Here's how the part is built. I have some questions about the finished solid (model axes, mm). Give positions to 0.01 mm unless a question says otherwise; leave off trailing zeros. Loops run counter-clockwise (first coordinate to the right, second up) from the corner with the lowest first, then second, coordinate; pieces in that order, holes last. Notation, with made-up numbers: (82.25, 13) - (98.25, 13) arc R20 cw to (98.25, 47) - close; hole circle Ø7 at (54, -13). An arc over 180 degrees is marked (long way). Return JSON: item names as keys, results as strings. Group by question number.
(1) If we section it at D-D (z = -49.48): Please give me the cut outline in (x, y).
(2) For P1, Ø2, axis at x = -75.5, y = 3, coming from the -Z side; P2, Ø1, axis at x = 34.5, y = 2.5, coming from the -Z side; P3, Ø6.5, axis at x = 0, z = -49.48, coming from the +Y side; P4, Ø2, axis at x = 47, y = 1, coming from the -Z side, each with a flat end and sliding along its axis, tell me the tip position at first contact or that it passes through.
(3) If we section it at C-C (y = 2.15): Please give me the cut outline in (x, z), then the cut area to 3 significant figures.
(4) If we section it at A-A (x = 0): Please give me the cut outline in (y, z).
(5) If we section it at B-B (z = 24.74): Please give me the cut outline in (x, y), then the cut area to 3 significant figures.
(6) I need wall thicknesses on probe 1 along X at (y, z) = (0.9, 24.74); probe 2 along Z at (x, y) = (47.5, 1.5); probe 3 along X at (y, z) = (1.4, -49.48). Which ranges of each line are inside material? Lowest first, please. Write a range as [from, to].
```python
from build123d import *

# Parameters (mm, degrees)
ESBO_O1_R                = 105
RESSALTO_EXTRUS_O1_DEPTH = 4
CORTE_EXTRUS_O1_DEPTH    = 5
ESBO_O3_R                = 4
CORTE_EXTRUS_O2_DEPTH    = 5
CORTE_EXTRUS_O3_REACH    = 6
ESBO_O4_W                = 15
ESBO_O4_H                = 10


with BuildPart() as part:
    # Esboço1 → Ressalto-extrusão1 (new body)
    with BuildSketch(Plane(origin=(0, 0, 0), x_dir=(1, 0, 0), z_dir=(0, 1, 0))):
        Circle(ESBO_O1_R)
    extrude(amount=RESSALTO_EXTRUS_O1_DEPTH)

    # Esboço2 → Corte-extrusão1 (cut, through all)
    with BuildSketch(Plane(origin=(0, 4, 0), x_dir=(1, 0, 0), z_dir=(0, 1, 0))):
        with BuildLine():
            Line((-6.077686218, -34.468271355), (-11.634427904, -65.982119452))
            ThreePointArc((-11.634427904, -65.982119452), (0, -67), (11.634427904, -65.982119452))
            Line((11.634427904, -65.982119452), (6.077686218, -34.468271355))
            ThreePointArc((6.077686218, -34.468271355), (0, -35), (-6.077686218, -34.468271355))
        make_face()
    extrude(amount=-CORTE_EXTRUS_O1_DEPTH, mode=Mode.SUBTRACT)

    # Esboço3 → Corte-extrusão2 (cut, through all)
    with BuildSketch(Plane(origin=(0, 4, 0), x_dir=(1, 0, 0), z_dir=(0, 1, 0))):
        with Locations((42.850936979, -24.74)):
            Circle(ESBO_O3_R)
        with Locations((0, 49.48)):
            Circle(ESBO_O3_R)
        with Locations((-42.850936979, -24.74)):
            Circle(ESBO_O3_R)
    extrude(amount=-CORTE_EXTRUS_O2_DEPTH, mode=Mode.SUBTRACT)

    # Esboço4 → Corte-extrusão3 (cut, up to next)
    with BuildSketch(Plane(origin=(0, 4, 0), x_dir=(1, 0, 0), z_dir=(0, 1, 0)), mode=Mode.PRIVATE) as corte_extrus_o3_sk1:
        with Locations((47.5, 29.48)):
            Rectangle(ESBO_O4_W, ESBO_O4_H)
    corte_extrus_o3_tool1 = extrude(corte_extrus_o3_sk1.sketch, amount=-CORTE_EXTRUS_O3_REACH, mode=Mode.PRIVATE) & part.part
    add(corte_extrus_o3_tool1.solids().sort_by_distance((47.5, 4, -29.48))[0], mode=Mode.SUBTRACT)


solid = part.part
```
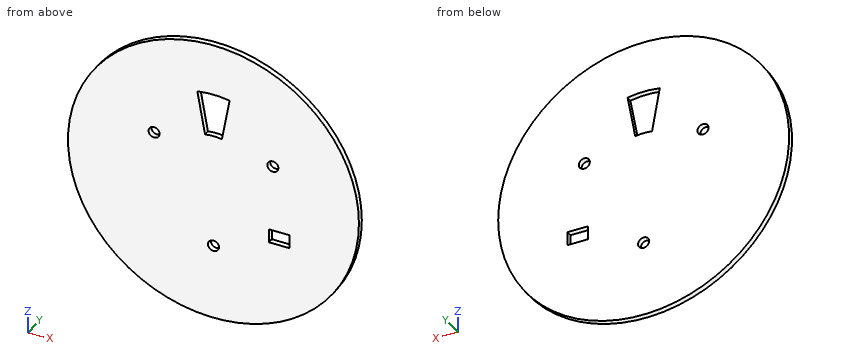
Values:
{
 "1": {"outline": "(-92.61, 0) - (-4, 0) - (-4, 4) - (-92.61, 4) - close; (4, 0) - (92.61, 0) - (92.61, 4) - (4, 4) - close"},
 "2": {"P1": "z = -73.99", "P2": "z = -99.34", "P3": "through", "P4": "z = -94.39"},
 "3": {"outline": "circle Ø210 at (0, 0); hole circle Ø8 at (-42.85, 24.74); hole (-11.63, 65.98) - (-6.08, 34.47) arc R35 cw to (6.08, 34.47) - (11.63, 65.98) arc R67 ccw to start; hole circle Ø8 at (0, -49.48); hole circle Ø8 at (42.85, 24.74); hole (40, -34.48) - (55, -34.48) - (55, -24.48) - (40, -24.48) - close", "area": "33,800 mm2"},
 "4": {"outline": "(0, -105) - (4, -105) - (4, -53.48) - (0, -53.48) - close; (0, -45.48) - (4, -45.48) - (4, 35) - (0, 35) - close; (0, 67) - (4, 67) - (4, 105) - (0, 105) - close"},
 "5": {"outline": "(-102.04, 0) - (-46.85, 0) - (-46.85, 4) - (-102.04, 4) - close; (-38.85, 0) - (38.85, 0) - (38.85, 4) - (-38.85, 4) - close; (46.85, 0) - (102.04, 0) - (102.04, 4) - (46.85, 4) - close", "area": "752 mm2"},
 "6": {"probe 1": "[-102.04, -46.85], [-38.85, 38.85], [46.85, 102.04]", "probe 2": "[-93.64, -34.48], [-24.48, 93.64]", "probe 3": "[-92.61, -4], [4, 92.61]"}
}
